Model file for the job. Use its own axes, mm. A direction names the side the tool comes from. Give positions to 0.01 mm unless a question says otherwise; leave off trailing zeros. Loops run counter-clockwise (first coordinate to the right, second up) from the corner with the lowest first, then second, coordinate; pieces in that order, holes last. Notation, with made-up numbers: M -17,85.25 L 37,85.25 A15 cw 37,96.25 Z; hole C 27.5,-38.5 d10. An arc over 180 degrees is marked long. Answer in a Markdown table with one row per item.
```python
from build123d import *

# Parameters (mm, degrees)
SKETCH_1_R          = 35
SKETCH_1_R_2        = 1.75
SKETCH_1_R_3        = 27.5
EXTRUDE_1_DEPTH     = 15
SKETCH_2_R          = 5
SKETCH_2_R_2        = 1.75
EXTRUDE_2_DEPTH     = 15
FILLET_1_R          = 3
SKETCH_3_R          = 5
CUT_EXTRUDE_1_DEPTH = 2
CUT_EXTRUDE_START   = -5
SKETCH_4_R          = 5
CUT_EXTRUDE_2_DEPTH = 5
FILLET_2_DEPTH      = 5
FILLET_3_R          = 1


with BuildPart() as part:
    # Эскиз1 → Бобышка-Вытянуть1 (new body)
    with BuildSketch(Plane(origin=(0, 0, 0), x_dir=(1, 0, 0), z_dir=(0, 1, 0))):
        with Locations(Location((0, 0, 0), (0, 0, 270))):
            Circle(SKETCH_1_R)
        with Locations(Location((-23.18, 22.0605, 0), (0, 0, 270))):
            Circle(SKETCH_1_R_2, mode=Mode.SUBTRACT)
        with Locations(Location((23.18, 22.0605, 0), (0, 0, 270))):
            Circle(SKETCH_1_R_2, mode=Mode.SUBTRACT)
        with Locations(Location((23.18, -22.0605, 0), (0, 0, 270))):
            Circle(SKETCH_1_R_2, mode=Mode.SUBTRACT)
        with Locations(Location((-23.18, -22.0605, 0), (0, 0, 270))):
            Circle(SKETCH_1_R_2, mode=Mode.SUBTRACT)
        with Locations(Location((0, 0, 0), (0, 0, 270))):
            Circle(SKETCH_1_R_3, mode=Mode.SUBTRACT)
    extrude(amount=EXTRUDE_1_DEPTH)

    # Эскиз2 → Бобышка-Вытянуть2 (add)
    # profile 1 of 3: a face of its own
    with BuildSketch(Plane(origin=(0, 15, 0), x_dir=(1, 0, 0), z_dir=(0, 1, 0))):
        with Locations((-13.13, 22.741827103)):
            Circle(SKETCH_2_R)
        with Locations((-13.13, 22.741827103)):
            Circle(SKETCH_2_R_2, mode=Mode.SUBTRACT)
    # profile 2 of 3: a face of its own
    with BuildSketch(Plane(origin=(0, 15, 0), x_dir=(1, 0, 0), z_dir=(0, 1, 0))):
        with Locations((26.26, 0)):
            Circle(SKETCH_2_R)
        with Locations((26.26, 0)):
            Circle(SKETCH_2_R_2, mode=Mode.SUBTRACT)
    # profile 3 of 3: a face of its own
    with BuildSketch(Plane(origin=(0, 15, 0), x_dir=(1, 0, 0), z_dir=(0, 1, 0))):
        with Locations((-13.13, -22.741827103)):
            Circle(SKETCH_2_R)
        with Locations((-13.13, -22.741827103)):
            Circle(SKETCH_2_R_2, mode=Mode.SUBTRACT)
    extrude(amount=-EXTRUDE_2_DEPTH)

    # Скругление1
    fillet_1_edges = [part.edges().sort_by_distance(p)[0] for p in [
        (27.053267327, 7.5, -4.936671647),
        (27.053267327, 7.5, 4.936671647),
        (-17.80191672, 7.5, -20.960480937),
        (-9.251350607, 7.5, -25.897152584),
        (-9.251350607, 7.5, 25.897152584),
        (-17.80191672, 7.5, 20.960480937),
    ]]
    fillet(fillet_1_edges, radius=FILLET_1_R)

    # Эскиз3 → Вырез-Вытянуть1 (cut)
    with BuildSketch(Plane(origin=(0, 15, 0), x_dir=(1, 0, 0), z_dir=(0, 1, 0))):
        with Locations((-23.18, 22.0605)):
            Circle(SKETCH_3_R)
        with Locations((23.18, 22.0605)):
            Circle(SKETCH_3_R)
        with Locations((23.18, -22.0605)):
            Circle(SKETCH_3_R)
        with Locations((-23.18, -22.0605)):
            Circle(SKETCH_3_R)
    extrude(amount=-CUT_EXTRUDE_1_DEPTH, mode=Mode.SUBTRACT)

    # Эскиз4 → Вырез-Вытянуть2 (cut)
    with BuildSketch(Plane.XZ.offset(CUT_EXTRUDE_START)):
        with Locations((-13.13, 22.741827103)):
            Circle(SKETCH_4_R)
        with Locations((26.26, 0)):
            Circle(SKETCH_4_R)
        with Locations((-13.13, -22.741827103)):
            Circle(SKETCH_4_R)
    extrude(amount=CUT_EXTRUDE_2_DEPTH, mode=Mode.SUBTRACT)

    # Скругление2: read off the stored shape, not the designer's step
    # Скругление2 outline → Скругление2 (cut)
    with BuildSketch(Plane(origin=(0, 0, 0), x_dir=(1, 0, 0), z_dir=(0, 1, 0))):
        with BuildLine():
            ThreePointArc((-16.249088608, 18.83397779), (-17.48691602, 20.288812061), (-18.08884989, 22.101664805))
            ThreePointArc((-18.08884989, 22.101664805), (-18.38244619, 20.372795331), (-19.592350799, 19.103417814))
            ThreePointArc((-19.592350799, 19.103417814), (-17.87954729, 19.479572812), (-16.249088608, 18.83397779))
        make_face()
        with BuildLine():
            ThreePointArc((-6.747869727, 26.519182418), (-8.452135208, 26.10606305), (-10.096178242, 26.716235932))
            ThreePointArc((-10.096178242, 26.716235932), (-8.827168648, 25.288519537), (-8.186158917, 23.489112418))
            ThreePointArc((-8.186158917, 23.489112418), (-7.930031265, 25.223928567), (-6.747869727, 26.519182418))
        make_face()
        with BuildLine():
            ThreePointArc((24.435247525, 4.655134628), (26.314084667, 4.999707476), (28.185028132, 4.614571128))
            ThreePointArc((28.185028132, 4.614571128), (26.834581398, 5.733267719), (26.340220525, 7.415764604))
            ThreePointArc((26.340220525, 7.415764604), (25.809578555, 5.744355755), (24.435247525, 4.655134628))
        make_face()
        with BuildLine():
            ThreePointArc((26.340220525, -7.415764604), (26.834581398, -5.733267719), (28.185028132, -4.614571128))
            ThreePointArc((28.185028132, -4.614571128), (26.314084667, -4.999707476), (24.435247525, -4.655134628))
            ThreePointArc((24.435247525, -4.655134628), (25.809578555, -5.744355755), (26.340220525, -7.415764604))
        make_face()
        with BuildLine():
            ThreePointArc((-8.186158917, -23.489112418), (-8.827168648, -25.288519537), (-10.096178242, -26.716235932))
            ThreePointArc((-10.096178242, -26.716235932), (-8.452135208, -26.10606305), (-6.747869727, -26.519182418))
            ThreePointArc((-6.747869727, -26.519182418), (-7.930031265, -25.223928567), (-8.186158917, -23.489112418))
        make_face()
        with BuildLine():
            ThreePointArc((-19.592350799, -19.103417814), (-18.38244619, -20.372795331), (-18.08884989, -22.101664805))
            ThreePointArc((-18.08884989, -22.101664805), (-17.48691602, -20.288812061), (-16.249088608, -18.83397779))
            ThreePointArc((-16.249088608, -18.83397779), (-17.87954729, -19.479572812), (-19.592350799, -19.103417814))
        make_face()
    extrude(amount=FILLET_2_DEPTH, mode=Mode.SUBTRACT)

    # Скругление3
    fillet_3_edges = [part.edges().sort_by_distance(p)[0] for p in [
        (-18.967333591, 14, -19.36727856),
        (-18.967333591, 14, 19.36727856),
        (21.259108635, 14, 17.444205342),
        (18.474346617, 14, 20.370285149),
        (22.293687033, 14, -26.981317953),
        (28.050957484, 14, -20.931884393),
        (-21.259108635, 14, 17.444205342),
        (-28.050957484, 14, 20.931884393),
        (-22.293687033, 14, 26.981317953),
        (22.293687033, 14, 26.981317953),
        (28.050957484, 14, 20.931884393),
        (21.259108635, 14, -17.444205342),
        (18.474346617, 14, -20.370285149),
        (-21.259108635, 14, -17.444205342),
        (-22.293687033, 14, -26.981317953),
        (-28.050957484, 14, -20.931884393),
    ]]
    fillet(fillet_3_edges, radius=FILLET_3_R)


solid = part.part
```
(1) Wall check: L1, parallel to Z at x = 23.18, y = 9.25; L2, parallel to Z at x = 0, y = 10.5; L3, parallel to X at y = 14, z = 23.5. Give the ranges that are in metal, low to high.
Established:
| item | result |
|---|---|
| L1 | z = -26.22 to -23.81, -20.31 to -14.8, -3.94 to 3.94, 14.8 to 20.31, 23.81 to 26.22 |
| L2 | z = -35 to -27.5, 27.5 to 35 |
| L3 | x = -18.39 to -14.28, -11.55 to -8.19, 14.28 to 18.39 |
(2) Saw through at C-C, the plane y = 4. Count the separate pieces of the cut face and the enclosed holes in it, and give its area (3 significant figures).
Established:
| item | result |
|---|---|
| separate pieces | 1 |
| enclosed holes | 5 |
| area | 1,350 mm2 |
(3) Saw through at B-B, the plane z = 0. Give the cut face in (x, y).
Established:
| item | result |
|---|---|
| outline | M -35,0 L -27.5,0 L -27.5,15 L -35,15 Z; M 21.26,5 L 24.51,5 L 24.51,15 L 21.26,15 Z; M 27.5,5 L 31.26,5 L 31.26,0 L 35,0 L 35,15 L 27.5,15 Z |
(4) Flat gauge pins, fed straight in: P1, Ø4, axis at x = 23.18, z = -22.06, coming from the +Y side; P2, Ø1, axis at x = -19, y = 4, coming from the +Z side; P3, Ø8, axis at x = 25, z = 1, coming from the -Y side; P4, Ø3, axis at x = 23.18, z = 22.06, coming from the +Y side. Where does each tip first touch, or does it go through?
Established:
| item | result |
|---|---|
| P1 | stops at y = 13 |
| P2 | stops at z = 29.71 |
| P3 | stops at y = 5 |
| P4 | passes through |
(5) Mould opens along Z. For faces 1 (the cylindrical face through (-13.735, 9.93, -23.825)), 2 (the flat face through (18, 0, -21)), 3 (the cylindrical face through (-25.71, 14.01, 17.75)) say: pulls with the +Z half, pulls with the -Z half, needs draft (parallel to the pull), parting line crosses it, or undercut.
Established:
| item | result |
|---|---|
| face 1 | undercut |
| face 2 | needs draft |
| face 3 | pulls with the +Z half |
(6) Which spindle directions (+Z, -Z, +X, -X, +Y, -Y) get a long thin tool onto all of the face, cutting with end or side? Do faces 4 (the cylindrical face through (19.03, 14.01, -24.85)), 5 (the cylindrical face through (13.5, 7.4, 23.96)), 6 (the cylindrical face through (31.26, 2.54, -0.08)), 7 (the flat face through (-22, 13, 20)). Say none if no direction does.
Established:
| item | result |
|---|---|
| face 4 | +X, +Y |
| face 5 | +Y, -Y |
| face 6 | -Y |
| face 7 | +Y |
(7) Saw through at A-A, the plane x = 0. Give the cut face in (y, z), and give its area (3 significant figures).
Established:
| item | result |
|---|---|
| outline | M 0,-35 L 15,-35 L 15,-27.5 L 0,-27.5 Z; M 0,27.5 L 15,27.5 L 15,35 L 0,35 Z |
| area | 225 mm2 |
